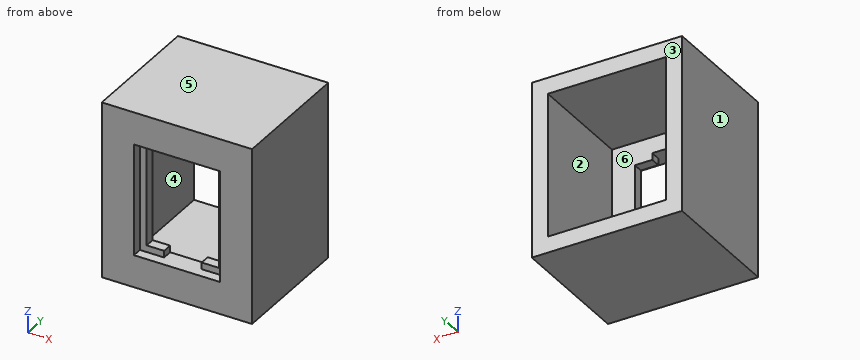
from build123d import *

# Parameters (mm, degrees)
SKETCH1_W           = 22
SKETCH1_H           = 26.75
SKETCH1_W_2         = 16
SKETCH1_H_2         = 20.75
BOSS_EXTRUDE2_DEPTH = 3.75
BOSS_EXTRUDE3_DEPTH = 1.875
SKETCH3_W           = 22
SKETCH3_H           = 3.75
BOSS_EXTRUDE4_DEPTH = 3
SKETCH4_W           = 29.75
SKETCH4_H           = 3.75
BOSS_EXTRUDE5_DEPTH = 3
SKETCH5_W           = 25
SKETCH5_H           = 3.75
BOSS_EXTRUDE6_DEPTH = 3
SKETCH6_W           = 32.75
SKETCH6_H           = 3.75
BOSS_EXTRUDE7_DEPTH = 3
SKETCH7_W           = 28
SKETCH7_H           = 32.75
SKETCH7_W_2         = 22
SKETCH7_H_2         = 26.75
BOSS_EXTRUDE8_DEPTH = 20


with BuildPart() as part:
    # Sketch1 → Boss-Extrude2 (new body)
    with BuildSketch(Plane(origin=(0, 0, 0), x_dir=(1, 0, 0), z_dir=(0, 1, 0))):
        with Locations((-47.484558715, -14.904779002)):
            Rectangle(SKETCH1_W, SKETCH1_H)
        with Locations((-47.484558715, -14.904779002)):
            Rectangle(SKETCH1_W_2, SKETCH1_H_2, mode=Mode.SUBTRACT)
    extrude(amount=BOSS_EXTRUDE2_DEPTH)

    # Sketch2 → Boss-Extrude3 (add)
    with BuildSketch(Plane(origin=(0, 3.75, 0), x_dir=(1, 0, 0), z_dir=(0, 1, 0))):
        Polygon((-50.984558715, -25.279779002), (-55.484558715, -25.279779002), (-55.484558715, -4.529779002), (-50.984558715, -4.529779002), (-50.984558715, -5.779779002), (-54.234558715, -5.779779002), (-54.234558715, -24.029779002), (-50.984558715, -24.029779002), align=None)
        Polygon((-43.984558715, -4.529779002), (-39.484558715, -4.529779002), (-39.484558715, -25.279779002), (-43.984558715, -25.279779002), (-43.984558715, -24.029779002), (-40.734558715, -24.029779002), (-40.734558715, -5.779779002), (-43.984558715, -5.779779002), align=None)
    extrude(amount=-BOSS_EXTRUDE3_DEPTH)

    # Sketch3 → Boss-Extrude4 (add)
    with BuildSketch(Plane(origin=(0, 0, 1.529779002), x_dir=(-1, 0, 0), z_dir=(0, 0, -1))):
        with Locations((47.484558715, 1.875)):
            Rectangle(SKETCH3_W, SKETCH3_H)
    extrude(amount=BOSS_EXTRUDE4_DEPTH)

    # Sketch4 → Boss-Extrude5 (add)
    with BuildSketch(Plane.ZY.offset(58.484558715)):
        with Locations((13.404779002, 1.875)):
            Rectangle(SKETCH4_W, SKETCH4_H)
    extrude(amount=BOSS_EXTRUDE5_DEPTH)

    # Sketch5 → Boss-Extrude6 (add)
    with BuildSketch(Plane.XY.offset(28.279779002)):
        with Locations((-48.984558715, 1.875)):
            Rectangle(SKETCH5_W, SKETCH5_H)
    extrude(amount=BOSS_EXTRUDE6_DEPTH)

    # Sketch6 → Boss-Extrude7 (add)
    with BuildSketch(Plane(origin=(-36.484558715, 0, 0), x_dir=(0, 0, -1), z_dir=(1, 0, 0))):
        with Locations((-14.904779002, 1.875)):
            Rectangle(SKETCH6_W, SKETCH6_H)
    extrude(amount=BOSS_EXTRUDE7_DEPTH)

    # Sketch7 → Boss-Extrude8 (add)
    with BuildSketch(Plane(origin=(0, 3.75, 0), x_dir=(1, 0, 0), z_dir=(0, 1, 0))):
        with Locations((-47.484558715, -14.904779002)):
            Rectangle(SKETCH7_W, SKETCH7_H)
        with Locations((-47.484558715, -14.904779002)):
            Rectangle(SKETCH7_W_2, SKETCH7_H_2, mode=Mode.SUBTRACT)
    extrude(amount=BOSS_EXTRUDE8_DEPTH)


solid = part.part
Design review of the part built by this model. Coordinates are the model's own, in mm. Face numbers are marked on the shaded views. A direction names the side the tool comes from. Round coordinates to 2 decimals unless told otherwise and drop trailing zeros. Loops run counter-clockwise (first coordinate to the right, second up) from the corner with the lowest first, then second, coordinate; pieces in that order, holes last. Notation, with made-up numbers: (-32, 27) -> (23, 27) arc R30 cw to (23, 63) -> close; hole circle Ø10 at (46.5, -13.75). An arc over 180 degrees is marked (long way). Use one line per item in the form item = value. Start each with the question number.
Q1. For pin 1 Ø12 at (x, z) = (-50.5, 14) entering from +Y; pin 2 Ø1.3 at (x, z) = (-41, 11.5) entering from -Y (3 decimals); pin 3 Ø1 at (x, z) = (-42.5, 16.5) entering from -Y, all flat-tipped, find the tip position at first contact; note any pin that passes through.
Q2. We need section B-B on x = -43.5. Give the boundary of the cut face in (y, z) (3 decimals).
Q3. Draft analysis for pull direction Z (two halves, no side actions). For the marked faces 3, 4, 5 and 6, state which applies: +Z half, -Z half, draft (parallel to the pull), parting line (faces both ways), or undercut.
Q4. Machinability: for the marked faces 1 and 2, which of the approach directions +Z, -Z, +X, -X, +Y, -Y give a long, thin tool a straight path to every point of the face, cutting with its end or side? Answer none if there is none.
Q5. We need section D-D on z = 2. Give the boundary of the cut face in (x, y).
Q6. We need section A-A on y = 5.25. Give the boundary of the cut face in (x, z), then the cut area to 4 significant figures.
Q7. We need section C-C on z = 8.5. Give the boundary of the cut face in (x, y) (3 decimals).
Q8. Wall thickness on line 1 along Z through (x, y) = (-39.25, 9.25); line 2 along X through (y, z) = (16.5, 23); line 3 along Z through (x, y) = (-40, 1.25): over which ranges is each line inside the solid? List them lowest first. Write a range as [from, to].
Calculated:
q1.pin_1 = 3.75
q1.pin_2 = 1.875
q1.pin_3 = through
q2.outline = (0, -1.47) -> (23.75, -1.47) -> (23.75, 1.53) -> (3.75, 1.53) -> (3.75, 5.78) -> (1.875, 5.78) -> (1.875, 4.53) -> (0, 4.53) -> close; (0, 25.28) -> (1.875, 25.28) -> (1.875, 24.03) -> (3.75, 24.03) -> (3.75, 28.28) -> (23.75, 28.28) -> (23.75, 31.28) -> (0, 31.28) -> close
q3.face_3 = draft
q3.face_4 = undercut
q3.face_5 = +Z half
q3.face_6 = undercut
q4.face_1 = +Z, -Z, -X, +Y, -Y
q4.face_2 = +Y
q5.outline = (-61.48, 0) -> (-33.48, 0) -> (-33.48, 23.75) -> (-36.48, 23.75) -> (-36.48, 3.75) -> (-58.48, 3.75) -> (-58.48, 23.75) -> (-61.48, 23.75) -> close
q6.outline = (-61.48, -1.47) -> (-33.48, -1.47) -> (-33.48, 31.28) -> (-61.48, 31.28) -> close; hole (-58.48, 1.53) -> (-36.48, 1.53) -> (-36.48, 28.28) -> (-58.48, 28.28) -> close
q6.area = 328.5 mm²
q7.outline = (-61.485, 0) -> (-55.485, 0) -> (-55.485, 1.875) -> (-54.235, 1.875) -> (-54.235, 3.75) -> (-58.485, 3.75) -> (-58.485, 23.75) -> (-61.485, 23.75) -> close; (-40.735, 1.875) -> (-39.485, 1.875) -> (-39.485, 0) -> (-33.485, 0) -> (-33.485, 23.75) -> (-36.485, 23.75) -> (-36.485, 3.75) -> (-40.735, 3.75) -> close
q8.line_1 = [-1.47, 1.53], [28.28, 31.28]
q8.line_2 = [-61.48, -58.48], [-36.48, -33.48]
q8.line_3 = [-1.47, 4.53], [25.28, 31.28]
